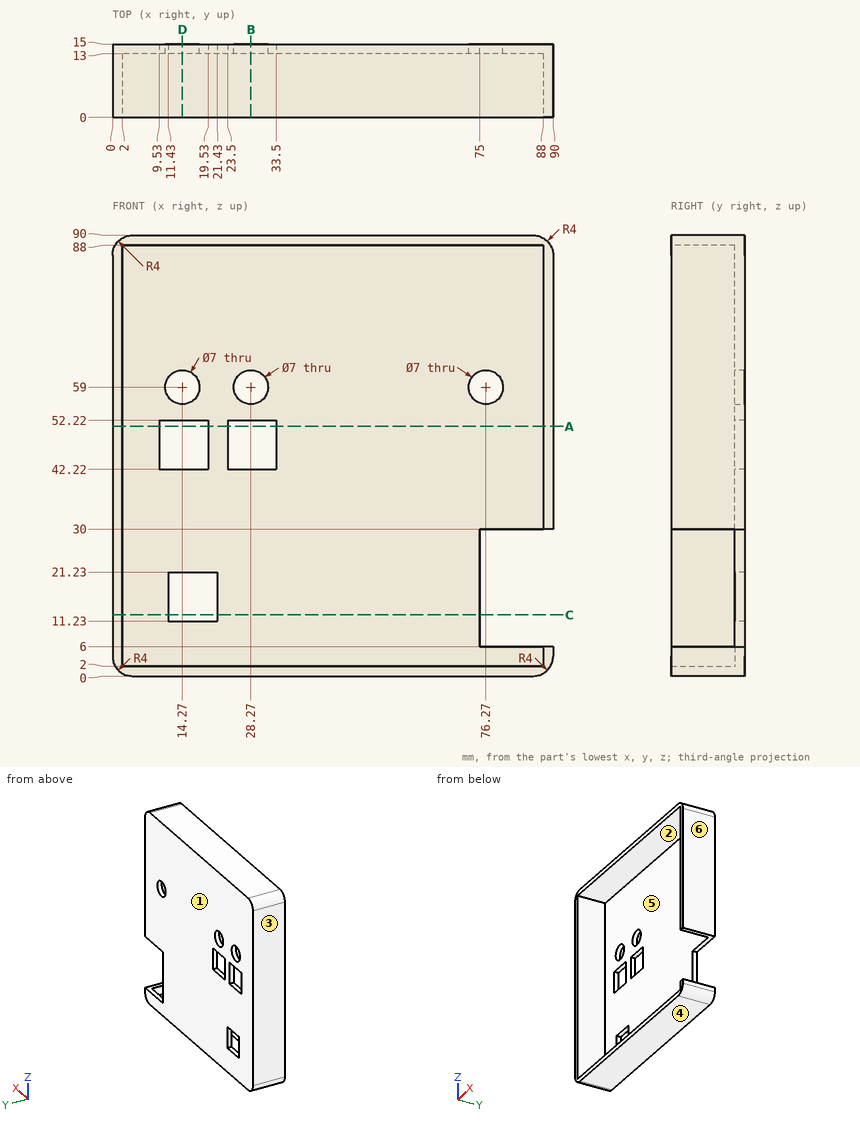
Design review of the part shown in the three views and the two pictorial views. Dimensions are in mm from the part's minimum x, y and z. A direction names the side the tool comes from. Coordinates: 2 decimals unless noted, no trailing zeros. Order: outer loops, then holes, each group sorted by start corner. A loop starts at its lowest first (then second) coordinate and runs counter-clockwise, first axis right, second up.
Item 1: For line 1 (X direction, y = 14, z = 59); line 2 (Z direction, x = 17, y = 11.5); line 3 (X direction, y = 13.5, z = 44.5), list the stretches that pass through material, from the lowest coordinate up.
Item 2: Take a section at C-C, the plane z = 12.5. Write out the cut boundary in (x, y).
Item 3: The part is to be moulded in two halves that separate along X. For the marked faces 3, 4, 5 and 6, say which applies: pulls with the +X half, pulls with the -X half, needs draft (parallel to the pull), parting line crosses it, or undercut.
Item 4: Take a section at D-D, the plane x = 14.27. Write out the cut boundary in (y, z).
Item 5: Take a section at A-A, the plane z = 51. Write out the cut boundary in (x, y).
Item 6: For pin 1 Ø1.5 at (x, y) = (59.5, 5) entering from -Z; pin 2 Ø6 at (x, z) = (15.5, 18.5) entering from -Y, all flat-tipped, find the tip position at first contact; note any pin that passes through.
Item 7: For the marked faces 1 and 2, list the 3-axis set-ups (+Z, -Z, +X, -X, +Y, -Y) from which the entire face can be reached by the end or side of a thin tool; tool diameter is ignored.
Item 8: Take a section at B-B, the plane x = 28.27. Write out the cut boundary in (y, z).
The answers:
1. line 1: x = 0 to 10.77, 17.77 to 24.77, 31.77 to 72.77, 79.77 to 90
1. line 2: z = 0 to 2, 88 to 90
1. line 3: x = 0 to 9.53, 19.53 to 23.5, 33.5 to 90
2. outline: (0, 0) - (2, 0) - (2, 13) - (11.43, 13) - (11.43, 15) - (0, 15) - close; (21.43, 13) - (75, 13) - (75, 15) - (21.43, 15) - close
3. face 3: pulls with the -X half
3. face 4: needs draft
3. face 5: undercut
3. face 6: pulls with the +X half
4. outline: (0, 0) - (15, 0) - (15, 11.23) - (13, 11.23) - (13, 2) - (0, 2) - close; (0, 88) - (13, 88) - (13, 62.5) - (15, 62.5) - (15, 90) - (0, 90) - close; (13, 21.23) - (15, 21.23) - (15, 42.22) - (13, 42.22) - close; (13, 52.22) - (15, 52.22) - (15, 55.5) - (13, 55.5) - close
5. outline: (0, 0) - (2, 0) - (2, 13) - (9.53, 13) - (9.53, 15) - (0, 15) - close; (19.53, 13) - (23.5, 13) - (23.5, 15) - (19.53, 15) - close; (33.5, 13) - (88, 13) - (88, 0) - (90, 0) - (90, 15) - (33.5, 15) - close
6. pin 1: stops at z = 0
6. pin 2: stops at y = 13
7. face 1: +Z, -Z, +X, -X, +Y
7. face 2: -Y
8. outline: (0, 0) - (15, 0) - (15, 42.22) - (13, 42.22) - (13, 2) - (0, 2) - close; (0, 88) - (13, 88) - (13, 62.5) - (15, 62.5) - (15, 90) - (0, 90) - close; (13, 52.22) - (15, 52.22) - (15, 55.5) - (13, 55.5) - close
